```python
from build123d import *

# Parameters (mm, degrees)
SKETCH1_W               = 120
SKETCH1_H               = 50
BOSS_EXTRUDE1_DEPTH     = 6
SKETCH2_W               = 20
SKETCH2_H               = 6
BOSS_EXTRUDE2_DEPTH     = 35
SKETCH3_W               = 20
SKETCH3_H               = 6
BOSS_EXTRUDE3_DEPTH     = 35
CUT_EXTRUDE1_DEPTH      = 83.006097334
CUT_EXTRUDE1_DEPTH_BACK = 83.006097334
SKETCH4_R               = 2.75


with BuildPart() as part:
    # Sketch1 → Boss-Extrude1 (new body)
    with BuildSketch(Plane(origin=(0, 0, 0), x_dir=(1, 0, 0), z_dir=(0, 1, 0))):
        Rectangle(SKETCH1_W, SKETCH1_H)
    extrude(amount=BOSS_EXTRUDE1_DEPTH)

    # Sketch2 → Boss-Extrude2 (add)
    with BuildSketch(Plane(origin=(0, 6, 0), x_dir=(1, 0, 0), z_dir=(0, 1, 0))):
        with Locations((-35, -10)):
            Rectangle(SKETCH2_W, SKETCH2_H)
    extrude(amount=BOSS_EXTRUDE2_DEPTH)

    # Sketch3 → Boss-Extrude3 (add)
    with BuildSketch(Plane(origin=(0, 6, 0), x_dir=(1, 0, 0), z_dir=(0, 1, 0))):
        with Locations((-35, 10)):
            Rectangle(SKETCH3_W, SKETCH3_H)
    extrude(amount=BOSS_EXTRUDE3_DEPTH)

    # Sketch4 → Cut-Extrude1 (cut, two sides: drawn at the far end of the back side and taken through both)
    with BuildSketch(Plane.XY.offset(13).offset(-CUT_EXTRUDE1_DEPTH_BACK)):
        with Locations((-35, 31)):
            Circle(SKETCH4_R)
    extrude(amount=CUT_EXTRUDE1_DEPTH + CUT_EXTRUDE1_DEPTH_BACK, mode=Mode.SUBTRACT)


solid = part.part
```
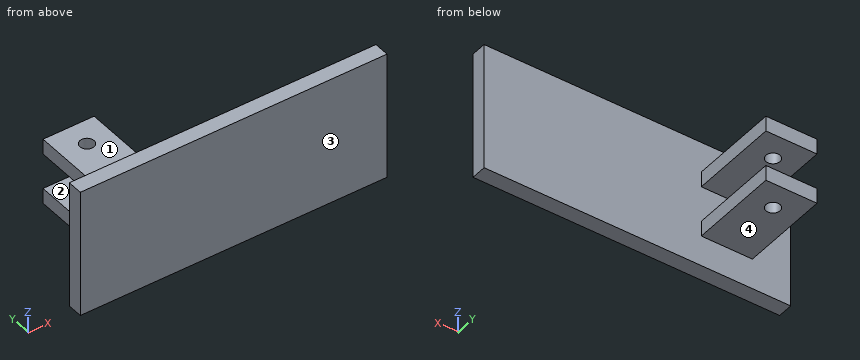
Can you work these out from the model? Positions are in its coordinate system, mm. Face numbers are marked on the shaded views. Coordinates: 2 decimals unless noted, no trailing zeros. Write each loop counter-clockwise with the first axis right and the second up, starting at its lowest first coordinate (ties: lowest second). Pieces come first, ordered by that corner, then holes. Notation, with made-up numbers: M -15,9 L 29,9 A7 ccw 29,18 Z; hole C -5.75,-9 d1. An arc over 180 degrees is marked long. Answer as CSV lines item,"result".
Item 1: Imagine slicing it at B-B on y = 31. List the corners of the cut face in (x, z) for me.
Geometry results:
outline,"M -45,-13 L -37.75,-13 L -37.75,-7 L -45,-7 Z; M -45,7 L -37.75,7 L -37.75,13 L -45,13 Z; M -32.25,-13 L -25,-13 L -25,-7 L -32.25,-7 Z; M -32.25,7 L -25,7 L -25,13 L -32.25,13 Z"
Item 2: We'd pull the mould along Z, two halves only. Please class the marked faces 1, 2, 3 and 4: +Z half, -Z half, draft (parallel to the pull), parting line (faces both ways), or undercut.
Geometry results:
face 1,"+Z half"
face 2,"undercut"
face 3,"draft"
face 4,"-Z half"
Item 3: Imagine slicing it at A-A on y = 15.5. List the corners of the cut face in (x, z) for me, plus the area to 3 significant figures.
Geometry results:
outline,"M -45,-13 L -25,-13 L -25,-7 L -45,-7 Z; M -45,7 L -25,7 L -25,13 L -45,13 Z"
area,"240 mm2"
Item 4: Please list where these lines run through material, in increasing order: line 1 along Y through (x, z) = (-35, -10.6); line 2 along X through (y, z) = (31, 9); line 3 along Z through (x, y) = (-40.5, 34).
Geometry results:
line 1,"y = 0 to 28.25, 33.75 to 41"
line 2,"x = -45 to -37.75, -32.25 to -25"
line 3,"z = -13 to -7, 7 to 13"
Item 5: Imagine slicing it at C-C on x = -35. List the corners of the cut face in (y, z) for me.
Geometry results:
outline,"M 0,-25 L 6,-25 L 6,-13 L 28.25,-13 L 28.25,-7 L 6,-7 L 6,7 L 28.25,7 L 28.25,13 L 6,13 L 6,25 L 0,25 Z; M 33.75,-13 L 41,-13 L 41,-7 L 33.75,-7 Z; M 33.75,7 L 41,7 L 41,13 L 33.75,13 Z"
Item 6: Imagine slicing it at D-D on z = 17. List the corners of the cut face in (x, y) for me, plus the area to 3 significant figures.
Geometry results:
outline,"M -60,0 L 60,0 L 60,6 L -60,6 Z"
area,"720 mm2"
Item 7: I'm going to push flat-ended pins straight in: P1, Ø22, axis at x = -33.5, y = 20.5, coming from the -Z side; P2, Ø5, axis at y = 26, z = -8.5, coming from the -X side; P3, Ø3, axis at y = 16.5, z = 10.5, coming from the +X side. Where does each tip first touch, or does it pass through?
Geometry results:
P1,"stops at z = -13"
P2,"stops at x = -45"
P3,"stops at x = -25"
